from build123d import *

# Parameters (mm, degrees)
SKETCH1_R            = 10
BOSS_EXTRUDE1_DEPTH  = 5
BOSS_EXTRUDE3_DEPTH  = 5
M3_CLEARANCE_HOLE1_D = 3.4
CIRPATTERN1_COUNT    = 3
FILLET1_R            = 10


with BuildPart() as part:
    # Sketch1 → Boss-Extrude1 (new body)
    with BuildSketch(Plane(origin=(0, 0, 0), x_dir=(1, 0, 0), z_dir=(0, 1, 0))):
        with BuildLine():
            Line((25, 7.5), (2.58079654, 12.230678199))
            ThreePointArc((2.58079654, 12.230678199), (-12.5, 0), (2.58079654, -12.230678199))
            Line((2.58079654, -12.230678199), (25, -7.5))
            Line((25, -7.5), (140, -7.5))
            ThreePointArc((140, -7.5), (147.5, 0), (140, 7.5))
            Line((140, 7.5), (25, 7.5))
        make_face()
        with Locations(Location((0, 0, 0), (0, 0, 270))):
            Circle(SKETCH1_R, mode=Mode.SUBTRACT)
        with BuildLine():
            ThreePointArc((142.348879749, -1.614082998), (137.15, 0), (142.348879749, 1.614082998))
            Line((142.348879749, 1.614082998), (142.348879749, -1.614082998))
        make_face(mode=Mode.SUBTRACT)
    extrude(amount=BOSS_EXTRUDE1_DEPTH)

    # Sketch2 → Boss-Extrude3 (add)
    with BuildSketch(Plane(origin=(0, 5, 0), x_dir=(1, 0, 0), z_dir=(0, 1, 0))):
        with BuildLine():
            ThreePointArc((-6.25, 10.825317547), (-4.412013956, 11.695474888), (-2.457258026, 12.256095748))
            Line((-2.457258026, 12.256095748), (-3.785898385, 14.557368355))
            ThreePointArc((-3.785898385, 14.557368355), (-9.25, 16.02146997), (-10.714101615, 10.557368355))
            Line((-10.714101615, 10.557368355), (-9.385461256, 8.256095748))
            ThreePointArc((-9.385461256, 8.256095748), (-7.922571384, 9.668653612), (-6.25, 10.825317547))
        make_face()
    boss_extrude3 = extrude(amount=-BOSS_EXTRUDE3_DEPTH)

    # M3 Clearance Hole1 (through all)
    with Locations(Plane(origin=(0, 5, 0), x_dir=(1, 0, 0), z_dir=(0, 1, 0))):
        with Locations((-7.25, 12.557368355)):
            m3_clearance_hole1 = Hole(M3_CLEARANCE_HOLE1_D / 2)

    # CirPattern1: Boss-Extrude3, M3 Clearance Hole1 ×3 about axis
    cirpattern1_axis = Axis((0, 0, 0), (0, 1, 0))
    add([boss_extrude3.rotate(cirpattern1_axis, i * 360 / CIRPATTERN1_COUNT) for i in range(1, CIRPATTERN1_COUNT)])
    add([m3_clearance_hole1.rotate(cirpattern1_axis, i * 360 / CIRPATTERN1_COUNT) for i in range(1, CIRPATTERN1_COUNT)], mode=Mode.SUBTRACT)

    # Fillet1
    fillet1_edges = [part.edges().sort_by_distance(p)[0] for p in [
        (-2.457258026, 2.5, 12.256095748),
        (-9.385461256, 2.5, 8.256095748),
        (-9.385461256, 2.5, -8.256095748),
        (-2.457258026, 2.5, -12.256095748),
        (25, 2.5, 7.5),
        (25, 2.5, -7.5),
    ]]
    fillet(fillet1_edges, radius=FILLET1_R)


solid = part.part
Design review of the part built by this model. Coordinates are the model's own, in mm. A direction names the side the tool comes from. Coordinates: 2 decimals unless noted, no trailing zeros. Loops run counter-clockwise (first coordinate to the right, second up) from the corner with the lowest first, then second, coordinate; pieces in that order, holes last.
Item 1: Draft analysis for pull direction Z (two halves, no side actions). For faces 1 (the flat face through (66, 0, 0)), 2 (the cylindrical face through (147.5, 2.46, 0.16)), 3 (the flat face through (142.349, 2, 0)), 4 (the cylindrical face through (137.15, 2.46, 0.1)), state which applies: pulls with the +Z half, pulls with the -Z half, needs draft (parallel to the pull), parting line crosses it, or undercut.
Completed:
face 1: needs draft
face 2: parting line crosses it
face 3: undercut
face 4: undercut
Item 2: Add section B-B (x = 69). Write out the cut boundary in (y, z), and give its area (3 significant figures).
Completed:
outline: (0, -7.5) - (5, -7.5) - (5, 7.5) - (0, 7.5) - close
area: 75.0 mm2
Item 3: Clearance check with flat-ended pins moving along their axes: pin 1 (2.5 mm diameter, centred on x = 14.5, z = 0, fed in from +Y); pin 2 (1.5 mm diameter, centred on x = 57, y = 3, fed in from -Z); pin 3 (3 mm diameter, centred on y = 1.5, z = -5, fed in from +X). State where each tip first meets the part, or that it passes through.
Completed:
pin 1: passes through
pin 2: stops at z = -7.5
pin 3: stops at x = 146.63
Item 4: Add section A-A (z = 0). Write out the cut boundary in (x, y).
Completed:
outline: (-12.5, 0) - (-10, 0) - (-10, 5) - (-12.5, 5) - close; (10, 0) - (12.8, 0) - (12.8, 5) - (10, 5) - close; (16.2, 0) - (137.15, 0) - (137.15, 5) - (16.2, 5) - close; (142.35, 0) - (147.5, 0) - (147.5, 5) - (142.35, 5) - close
Item 5: For faces 5 (the flat face through (82, 2, 7.5)), 6 (the flat face through (84, 2, -7.5)), 7 (the cylindrical face through (-12.5, 2.5, -0.1)), list the 3-axis set-ups (+Z, -Z, +X, -X, +Y, -Y) from which the entire face can be reached by the end or side of a thin tool; tool diameter is ignored.
Completed:
face 5: +Z, +X, +Y, -Y
face 6: -Z, +X, +Y, -Y
face 7: -X, +Y, -Y
Item 6: Wall thickness on L1, parallel to X at y = 0.3, z = -1; L2, parallel to Z at x = -7.25, y = 3.8; L3, parallel to X at y = 0.9, z = 0.5: over which ranges is each line inside the solid? List them lowest first.
Completed:
L1: x = -12.46 to -9.95, 9.95 to 13.13, 15.87 to 137.33, 142.35 to 147.43
L2: z = -16.56 to -14.26, -10.86 to -6.89, 6.89 to 10.86, 14.26 to 16.56
L3: x = -12.49 to -9.99, 9.99 to 12.88, 16.12 to 137.19, 142.35 to 147.48
Item 7: Add section C-C (y = 2.2). Give the number of separate pieces and of enclosed holes in the cut face, and give its area (3 significant figures).
Completed:
separate pieces: 1
enclosed holes: 5
area: 2,300 mm2
